The listing builds one solid part. Answer for the finished solid, in the listing's coordinates (mm). A direction names the side the tool comes from. Round coordinates to 2 decimals unless told otherwise and drop trailing zeros. Write each loop counter-clockwise with the first axis right and the second up, starting at its lowest first coordinate (ties: lowest second). Pieces come first, ordered by that corner, then holes.
(1) Each of these flat-tipped pins is pushed along its axis until it touches: pin 1 Ø5.5 at (x, z) = (-25.5, -15.5) entering from +Y; pin 2 Ø5 at (x, y) = (-23, 547.5) entering from +Z; pin 3 Ø9.5 at (x, z) = (-26.5, 106.5) entering from -Y. Where does it stop, or does it pass through?
(2) A cutting plane is placed at A-A, the plane x = -18.5. Give the vertices of the cut face in (y, z), and give its area (3 significant figures).
(3) A cutting plane is placed at B-B, the plane y = 164.5. Give the vertices of the cut face in (x, z).
(4) Find the intervals of material crossed by probe 1 along Y at (x, z) = (-30, 31); probe 2 along Z at (x, y) = (-21.25, 242), in increasing order.
(5) For faces 1 (the face through (-23, -8.589, 267)), 2 (the face through (-13.224, 269, 213)), 3 (the face through (-23, 501.392, -13)), 4 (the face through (-23, 275, 0)), 5 (the face through (-23, 1.012, 100)), determine the directions among +Z, -Z, +X, -X, +Y, -Y from which every point of the face is accessible in a straight line to the end or side of a thin tool.
(6) A cutting plane is placed at C-C, the plane z = 330.5. Give the vertices of the cut face in (x, y), and give its area (3 significant figures).
(7) The mould has two halves that part along Y. Classify faces 6 (the face through (-23, 554.173, 267)), 7 (the face through (-23, 44.192, -13)), 8 (the face through (-23, 544.572, 100)): +Y half, -Y half, draft (parallel to the pull), parting line (faces both ways), or undercut.
from build123d import *

# Parameters (mm, degrees)
F0_W      = 19.05
F0_H      = 543.56
F1_DEPTH  = 457.2
F2_W      = 19.05
F2_H      = 50.8
F3_DEPTH  = 19.1262
F4_W      = 19.05
F4_H      = 9.525
F5_DEPTH  = 25.4
F6_W      = 19.05
F6_H      = 50.8
F7_DEPTH  = 19.1262
F8_W      = 19.05
F8_H      = 9.525
F9_DEPTH  = 25.4
F10_W     = 19.05
F10_H     = 76.2
F11_DEPTH = 9.652
F12_DEPTH = 25.4


# Not quite as in the source:
# - a feature names something its author has since deleted; it is built from what else it names


with BuildPart() as f1:
    # F0 (on Top) → F1 (new body)
    with BuildSketch(Plane.XY):
        with Locations((-22.7488256648, 272.7919273724)):
            Rectangle(F0_W, F0_H)
    extrude(amount=F1_DEPTH)

    # F2 (on face) → F3 (join)
    with BuildSketch(Plane(origin=(0, 544.5719273724, 0), x_dir=(-1, 0, 0), z_dir=(0, 1, 0))):
        with Locations((22.7488256648, 228.6)):
            Rectangle(F2_W, F2_H)
    extrude(amount=F3_DEPTH)

    # F4 (on face) → F5 (join)
    with BuildSketch(Plane.XY.offset(254)):
        with Locations((-22.7488256648, 558.9356273724)):
            Rectangle(F4_W, F4_H)
    extrude(amount=F5_DEPTH)

    # F6 (on face) → F7 (join)
    with BuildSketch(Plane.XZ.offset(-1.0119273724)):
        with Locations((-22.7488256648, 228.6)):
            Rectangle(F6_W, F6_H)
    extrude(amount=F7_DEPTH)

    # F8 (on face) → F9 (join)
    with BuildSketch(Plane.XY.offset(254)):
        with Locations((-22.7488256648, -13.3517726276)):
            Rectangle(F8_W, F8_H)
    extrude(amount=F9_DEPTH)

    # F10 (on face) → F11 (join)
    with BuildSketch(Plane(origin=(0, 0, 0), x_dir=(1, 0, 0), z_dir=(0, 0, -1))):
        with Locations((-22.7488256648, -82.2919273724)):
            Rectangle(F10_W, F10_H)
        with Locations((-22.7488256648, -463.2919273724)):
            Rectangle(F10_W, F10_H)
    extrude(amount=F11_DEPTH)

    # F10 (on face) → F12 (join)
    with BuildSketch(Plane(origin=(0, 0, 0), x_dir=(1, 0, 0), z_dir=(0, 0, -1))):
        with Locations((-22.7488256648, -82.2919273724)):
            Rectangle(F10_W, F10_H)
        with Locations((-22.7488256648, -463.2919273724)):
            Rectangle(F10_W, F10_H)
    extrude(amount=F12_DEPTH)


solid = f1.part
Solutions:
1. pin 1: stops at y = 501.39
1. pin 2: stops at z = 254
1. pin 3: stops at y = 1.01
2. outline: (-18.11, 203.2) - (1.01, 203.2) - (1.01, 0) - (44.19, 0) - (44.19, -25.4) - (120.39, -25.4) - (120.39, 0) - (425.19, 0) - (425.19, -25.4) - (501.39, -25.4) - (501.39, 0) - (544.57, 0) - (544.57, 203.2) - (563.7, 203.2) - (563.7, 279.4) - (554.17, 279.4) - (554.17, 254) - (544.57, 254) - (544.57, 457.2) - (1.01, 457.2) - (1.01, 254) - (-8.59, 254) - (-8.59, 279.4) - (-18.11, 279.4) - close
2. area: 255,000 mm2
3. outline: (-32.27, 0) - (-13.22, 0) - (-13.22, 457.2) - (-32.27, 457.2) - close
4. probe 1: y = 1.01 to 544.57
4. probe 2: z = 0 to 457.2
5. face 1: +Z, +X, -X
5. face 2: +Z, -Z, +X, +Y, -Y
5. face 3: -Z, +X, -X, +Y
5. face 4: -Z, +X, -X
5. face 5: -Z, +X, -X, -Y
6. outline: (-32.27, 1.01) - (-13.22, 1.01) - (-13.22, 544.57) - (-32.27, 544.57) - close
6. area: 10,400 mm2
7. face 6: undercut
7. face 7: -Y half
7. face 8: +Y half
